```python
from build123d import *

# Parameters (mm, degrees)
SKICA1_R                 = 3
P_IDAT_VYSUNUT_M1_DEPTH  = 140
SKICA2_R                 = 4.5
P_IDAT_VYSUNUT_M2_DEPTH  = 7.5
ODEBRAT_VYSUNUT_M1_DEPTH = 4.5
ZKOSEN_1_SIZE            = 0.5


with BuildPart() as part:
    # Skica1 → Přidat vysunutím1 (new body)
    with BuildSketch(Plane.XY):
        Circle(SKICA1_R)
    extrude(amount=P_IDAT_VYSUNUT_M1_DEPTH)

    # Skica2 → Přidat vysunutím2 (add)
    with BuildSketch(Plane(origin=(0, 0, 0), x_dir=(-1, 0, 0), z_dir=(0, 0, -1))):
        Circle(SKICA2_R)
    extrude(amount=P_IDAT_VYSUNUT_M2_DEPTH)

    # Skica3 → Odebrat vysunutím1 (cut)
    with BuildSketch(Plane(origin=(0, 0, -7.5), x_dir=(-1, 0, 0), z_dir=(0, 0, -1))):
        Polygon((0, -2.771281292), (2.4, -1.385640646), (2.4, 1.385640646), (0, 2.771281292), (-2.4, 1.385640646), (-2.4, -1.385640646), align=None)
    extrude(amount=-ODEBRAT_VYSUNUT_M1_DEPTH, mode=Mode.SUBTRACT)

    # Zkosení1
    zkosen_1_edges = [part.edges().sort_by_distance(p)[0] for p in [
        (-3, 0, 140),
    ]]
    chamfer(zkosen_1_edges, length=ZKOSEN_1_SIZE)


solid = part.part
```
The model under review builds one solid part; all positions refer to its coordinate system, in mm. A direction names the side the tool comes from. Round coordinates to 2 decimals unless told otherwise and drop trailing zeros. Write each loop counter-clockwise with the first axis right and the second up, starting at its lowest first coordinate (ties: lowest second). Pieces come first, ordered by that corner, then holes. Notation, with made-up numbers: (47.25, 6.25) -> (53.25, 6.25) arc R15 ccw to (53.25, 24.25) -> close; hole circle Ø9 at (14.25, 66). An arc over 180 degrees is marked (long way). Use CSV: the item, a comma, the result in double quotes.
Q1. Mouldability with a two-part tool opening along Y and no side actions: class faces 1 (the cylindrical face through (-3, 0, 69)), 2 (the flat face through (1.217, -2.069, -5.281)), 3 (the flat face through (-1, -3, 0)) as released by +Y, released by -Y, zero draft, split by the parting line, or undercut.
Checks:
face 1,"split by the parting line"
face 2,"undercut"
face 3,"zero draft"
Q2. Consider section A-A (y = 0). Give the boundary of the cut face in (x, z).
Checks:
outline,"(-4.5, -7.5) -> (-2.4, -7.5) -> (-2.4, -3) -> (2.4, -3) -> (2.4, -7.5) -> (4.5, -7.5) -> (4.5, 0) -> (3, 0) -> (3, 139.5) -> (2.5, 140) -> (-2.5, 140) -> (-3, 139.5) -> (-3, 0) -> (-4.5, 0) -> close"
Q3. For faces 4 (the flat face through (1.18, 2.09, -5.28)), 5 (the flat face through (0, 0, 140)), list the 3-axis set-ups (+Z, -Z, +X, -X, +Y, -Y) from which the entire face can be reached by the end or side of a thin tool; tool diameter is ignored.
Checks:
face 4,"-Z"
face 5,"+Z, +X, -X, +Y, -Y"
Q4. Consider section B-B (z = 50.5). Give the boundary of the cut face in (x, y).
Checks:
outline,"circle Ø6 at (0, 0)"
Q5. To check wall thickness, follow probe 1 along Z at (x, y) = (1.75, 4); probe 2 along Z at (x, y) = (-0.5, 1.25); probe 3 along X at (y, z) = (2.75, 33.5). State the ranges of each line that lie inside material, in increasing order. Write a range as [from, to].
Checks:
probe 1,"[-7.5, 0]"
probe 2,"[-3, 140]"
probe 3,"[-1.2, 1.2]"
Q6. For pin 1 Ø3 at (y, z) = (-1, 69.5) entering from -X; pin 2 Ø2 at (x, z) = (-2.5, 111) entering from +Y; pin 3 Ø5 at (x, z) = (-3.5, 119) entering from -Y, all flat-tipped, find the tip position at first contact; note any pin that passes through.
Checks:
pin 1,"x = -3"
pin 2,"y = 2.6"
pin 3,"y = -2.83"
